Autodesk Inventor part; units mm, degrees
ref_plane "YZ Plane" through (0, 0, 0) normal (1, 0, 0) x (0, 1, 0)
ref_plane "XZ Plane" through (0, 0, 0) normal (0, 1, 0) x (-1, 0, 0)
ref_plane "XY Plane" through (0, 0, 0) normal (0, 0, 1) x (1, 0, 0)
sketch "Sketch1" plane through (0, 0, 0) normal (0, 1, 0) x (-1, 0, 0)
  circle A0 centre (0, 0) radius 19.05
  dimension "d0" = 38.1
extrude "Extrusion1" add sketch "Sketch1" along normal blind 1.5875
sketch "Sketch2" plane through (0, 1.5875, 0) normal (0, 1, 0) x (1, 0, 0)
  circle A0 centre (0, 0) radius 19.05
  circle A1 centre (0, 0) radius 17.4625
  dimension "d3" = 34.925
extrude "Extrusion2" add sketch "Sketch2" along normal blind 12.7 contours A1
sketch "Sketch3" plane through (0, 14.2875, 0) normal (0, 1, 0) x (1, 0, 0)
  circle A0 centre (0, 0) radius 17.4625
  circle A1 centre (0, 0) radius 7.9375
  dimension "d6" = 15.875
extrude "Extrusion3" cut sketch "Sketch3" against normal blind 2540 contours A1
properties part number "New Bearing"
Build history of the part. All positions in model axes, mm. A direction names the side the tool comes from. Round coordinates to 2 decimals unless told otherwise and drop trailing zeros. Order: outer loops, then holes, each group sorted by start corner. A loop starts at its lowest first (then second) coordinate and runs counter-clockwise, first axis right, second up. Notation, with made-up numbers: (85.25, 32) -> (106.25, 32) arc R22 cw to (106.25, 65) -> close; hole circle Ø9 at (-26.75, 8.5). An arc over 180 degrees is marked (long way). Answer in a Markdown table with one row per item.
1) Mould opens along Z. For faces 1 (the cylindrical face through (15.12, 0.78, 11.59)), 2 (the cylindrical face through (-1.72, 7.24, 7.75)), 3 (the flat face through (-17, 1.588, -6)) say: released by +Z, released by -Z, zero draft, split by the parting line, or undercut.
Values:
| item | result |
|---|---|
| face 1 | split by the parting line |
| face 2 | undercut |
| face 3 | zero draft |
2) Which spindle directions (+Z, -Z, +X, -X, +Y, -Y) get a long thin tool onto all of the face, cutting with end or side? Do faces 4 (the cylindrical face through (-13.858, 7.849, -10.626)), 5 (the flat face through (-8.2, 0, 0.3)). Say none if no direction does.
Values:
| item | result |
|---|---|
| face 4 | +Y |
| face 5 | +Z, -Z, +X, -X, -Y |
3) Pin check, flat tips, straight feed: P1, Ø1.5, axis at x = 9.5, y = 12.5, coming from the +Z side; P2, Ø8, axis at x = -3.5, y = 7, coming from the +Z side; P3, Ø12.5, axis at x = 0, z = 0, coming from the -Y side; P4, Ø1, axis at x = 9.5, y = 4, coming from the -Z side. Stop position of each tip, or through.
Values:
| item | result |
|---|---|
| P1 | z = 15.11 |
| P2 | z = 17.46 |
| P3 | through |
| P4 | z = -14.96 |
4) Wall check: L1, parallel to Z at x = 0, y = 6.5; L2, parallel to Y at x = -12.5, z = -14. Give the ranges that are in metal, low to high.
Values:
| item | result |
|---|---|
| L1 | -17.46 to -7.94, 7.94 to 17.46 |
| L2 | 0 to 1.59 |
5) Band-saw the part on A-A on z = 0. Give the cut face in (x, y), and give its area (3 significant figures).
Values:
| item | result |
|---|---|
| outline | (-19.05, 0) -> (-7.94, 0) -> (-7.94, 14.29) -> (-17.46, 14.29) -> (-17.46, 1.59) -> (-19.05, 1.59) -> close; (7.94, 0) -> (19.05, 0) -> (19.05, 1.59) -> (17.46, 1.59) -> (17.46, 14.29) -> (7.94, 14.29) -> close |
| area | 277 mm2 |
6) Band-saw the part on B-B on x = 0. Give the cut face in (y, z).
Values:
| item | result |
|---|---|
| outline | (0, -19.05) -> (1.59, -19.05) -> (1.59, -17.46) -> (14.29, -17.46) -> (14.29, -7.94) -> (0, -7.94) -> close; (0, 7.94) -> (14.29, 7.94) -> (14.29, 17.46) -> (1.59, 17.46) -> (1.59, 19.05) -> (0, 19.05) -> close |
7) Band-saw the part on C-C on y = 3. Give the cut face in (x, z) (1 decimal), and give its area (3 significant figures).
Values:
| item | result |
|---|---|
| outline | circle Ø34.9 at (0, 0); hole circle Ø15.9 at (0, 0) |
| area | 760 mm2 |
8) Band-saw the part on D-D on x = -16. Give the cut face in (y, z).
Values:
| item | result |
|---|---|
| outline | (0, -10.34) -> (1.59, -10.34) -> (1.59, -7) -> (14.29, -7) -> (14.29, 7) -> (1.59, 7) -> (1.59, 10.34) -> (0, 10.34) -> close |
